from build123d import *

# Parameters (mm, degrees)
F0_W     = 80
F0_H     = 19
F1_DEPTH = 19
F2_R     = 5.955
F2_R_2   = 5.25
F3_DEPTH = 19.001
F5_DEPTH = 19.001
F6_R     = 5
F7_DEPTH = 4.5


with BuildPart() as f1:
    # F0 (on Top) → F1 (new body)
    with BuildSketch(Plane.XY):
        Rectangle(F0_W, F0_H)
    extrude(amount=F1_DEPTH)

    # F2 (on face) → F3 (cut, through all)
    with BuildSketch(Plane(origin=(0, 9.5, 0), x_dir=(-1, 0, 0), z_dir=(0, 1, 0))):
        with Locations((20, 9.5)):
            Circle(F2_R)
        with Locations((-20, 9.5)):
            Circle(F2_R)
        with Locations((0, 9.5)):
            Circle(F2_R_2)
    extrude(amount=-F3_DEPTH, mode=Mode.SUBTRACT)

    # F4 (on face) → F5 (cut, through all)
    with BuildSketch(Plane.XY.offset(19)):
        with BuildLine():
            ThreePointArc((-27.45, 0), (-30, 2.55), (-32.55, 0))
            Line((-32.55, 0), (-27.45, 0))
        make_face()
        with BuildLine():
            ThreePointArc((32.55, 0), (30, 2.55), (27.45, 0))
            Line((27.45, 0), (32.55, 0))
        make_face()
        with BuildLine():
            Line((32.55, 0), (27.45, 0))
            ThreePointArc((27.45, 0), (30, -2.55), (32.55, 0))
        make_face()
        with BuildLine():
            ThreePointArc((12.55, 0), (10, 2.55), (7.45, 0))
            Line((7.45, 0), (12.55, 0))
        make_face()
        with BuildLine():
            Line((12.55, 0), (7.45, 0))
            ThreePointArc((7.45, 0), (10, -2.55), (12.55, 0))
        make_face()
        with BuildLine():
            ThreePointArc((-7.45, 0), (-10, 2.55), (-12.55, 0))
            Line((-12.55, 0), (-7.45, 0))
        make_face()
        with BuildLine():
            Line((-7.45, 0), (-12.55, 0))
            ThreePointArc((-12.55, 0), (-10, -2.55), (-7.45, 0))
        make_face()
        with BuildLine():
            Line((-27.45, 0), (-32.55, 0))
            ThreePointArc((-32.55, 0), (-30, -2.55), (-27.45, 0))
        make_face()
    extrude(amount=-F5_DEPTH, mode=Mode.SUBTRACT)

    # F6 (on face) → F7 (cut)
    with BuildSketch(Plane.XY.offset(19)):
        with Locations((-30, 0)):
            Circle(F6_R)
        with Locations((-10, 0)):
            Circle(F6_R)
        with Locations((10, 0)):
            Circle(F6_R)
        with Locations((30, 0)):
            Circle(F6_R)
    extrude(amount=-F7_DEPTH, mode=Mode.SUBTRACT)


solid = f1.part
CAD build for the part. Positions are in the model's coordinates, mm. A direction names the side the tool comes from. Round coordinates to 2 decimals unless told otherwise and drop trailing zeros. Loops run counter-clockwise (first coordinate to the right, second up) from the corner with the lowest first, then second, coordinate; pieces in that order, holes last. Notation, with made-up numbers: M 77,35 L 87,35 A9 ccw 87,43 Z; hole C -22.5,88 d1. An arc over 180 degrees is marked long. One line per question, with ' | ' between items. Start each with the question number.
Item 1: Pin check, flat tips, straight feed: pin 1 Ø3 at (x, y) = (-7.5, -5.5) entering from -Z; pin 2 Ø6.5 at (x, y) = (10, 0) entering from +Z. Stop position of each tip, or through.
Item 2: Which spindle directions (+Z, -Z, +X, -X, +Y, -Y) get a long thin tool onto all of the face, cutting with end or side? Do faces 5 (the cylindrical face through (-12.356, 0.977, 7.352)), 6 (the flat face through (-28, -2, 14.5)). Say none if no direction does.
Item 3: Two-plate mould, pull along Z, no slides. Class faces 1 (the flat face through (12, -2, 14.5)), 2 (the cylindrical face through (-27.452, -0.112, 7.352)), 3 (the cylindrical face through (0.683, 0.133, 14.705)), 4 (the cylindrical face through (-15.611, 0.133, 13.525)): pulls with the +Z half, pulls with the -Z half, needs draft (parallel to the pull), parting line crosses it, or undercut.
Item 4: Cut at B-B, the plane z = 8.25. Write the cut outline in (x, y), plus the area to 3 significant figures.
Item 5: Cut at C-C, the plane x = 20. Write the cut outline in (y, z) (3 decimals), plus the area to 3 significant figures.
Item 6: Wall check: line 1 (X direction, y = 2.25, z = 1); line 2 (Z direction, x = 0, y = -5.5); line 3 (Z direction, x = 20, y = -3) (3 decimals). Give the ranges that are in metal, low to high.
Item 7: Cut at A-A, the plane x = 10. Write the cut outline in (y, z), plus the area to 3 significant figures.
Item 8: Cut at D-D, the plane z = 12. Write the cut outline in (x, y).
Responses:
1) pin 1: stops at z = 0 | pin 2: stops at z = 14.5
2) face 5: +Z, -Z | face 6: +Z
3) face 1: pulls with the +Z half | face 2: needs draft | face 3: undercut | face 4: undercut
4) outline: M -40,-9.5 L -25.82,-9.5 L -25.82,9.5 L -40,9.5 Z; M -14.18,-9.5 L -5.1,-9.5 L -5.1,9.5 L -14.18,9.5 Z; M 5.1,-9.5 L 14.18,-9.5 L 14.18,9.5 L 5.1,9.5 Z; M 25.82,-9.5 L 40,-9.5 L 40,9.5 L 25.82,9.5 Z; hole C -30,0 d5.1; hole C -10,0 d5.1; hole C 10,0 d5.1; hole C 30,0 d5.1 | area: 802 mm²
5) outline: M -9.5,0 L 9.5,0 L 9.5,3.545 L -9.5,3.545 Z; M -9.5,15.455 L 9.5,15.455 L 9.5,19 L -9.5,19 Z | area: 135 mm²
6) line 1: x = -40 to -31.2, -28.8 to -11.2, -8.8 to 8.8, 11.2 to 28.8, 31.2 to 40 | line 2: z = 0 to 4.25, 14.75 to 19 | line 3: z = 0 to 3.545, 15.455 to 19
7) outline: M -9.5,0 L -2.55,0 L -2.55,14.5 L -5,14.5 L -5,19 L -9.5,19 Z; M 2.55,0 L 9.5,0 L 9.5,19 L 5,19 L 5,14.5 L 2.55,14.5 Z | area: 242 mm²
8) outline: M -40,-9.5 L -25.4,-9.5 L -25.4,9.5 L -40,9.5 Z; M -14.6,-9.5 L -4.62,-9.5 L -4.62,9.5 L -14.6,9.5 Z; M 4.62,-9.5 L 14.6,-9.5 L 14.6,9.5 L 4.62,9.5 Z; M 25.4,-9.5 L 40,-9.5 L 40,9.5 L 25.4,9.5 Z; hole C -30,0 d5.1; hole C -10,0 d5.1; hole C 10,0 d5.1; hole C 30,0 d5.1
